Geometry check sheet. Reference: drawing and pictorial views, mm from the part's lowest x, y, z. Give positions to 0.01 mm unless a question says otherwise; leave off trailing zeros. Write each loop counter-clockwise with the first axis right and the second up, starting at its lowest first coordinate (ties: lowest second). Pieces come first, ordered by that corner, then holes. Notation, with made-up numbers: M 68,-13.75 L 80,-13.75 A24 cw 80,21.25 Z; hole C 0.5,-7 d1. An arc over 180 degrees is marked long. Answer as a JSON object with one key per item and string values.
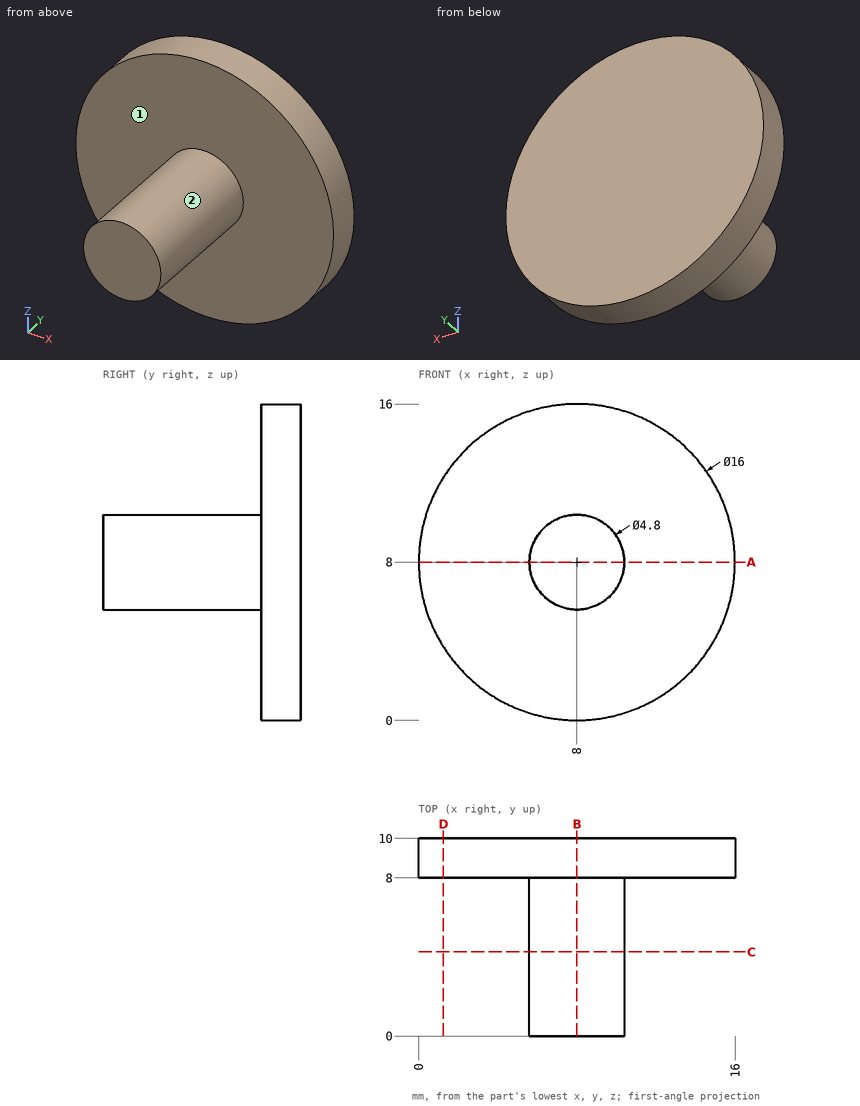
1) Release check for a two-part mould opening along X. For the marked faces 1 and 2 record: pulls with the +X half, pulls with the -X half, needs draft (parallel to the pull), parting line crosses it, or undercut.
Completed:
{"face 1": "needs draft", "face 2": "parting line crosses it"}
2) Section check C-C on y = 4.25. Record the boundary of the cut face in (x, z), and give its area (3 significant figures).
Completed:
{"outline": "C 8,8 d4.8", "area": "18.1 mm2"}
3) Go/stop test with flat-tipped pins: pin 1 (1.5 mm diameter, centred on x = 9, y = 6, fed in from -Z); pin 2 (3 mm diameter, centred on x = 2, z = 8, fed in from -Y); pin 3 (4 mm diameter, centred on x = 10, y = 6.5, fed in from -Z). Record where each tip stops, or that it passes through.
Completed:
{"pin 1": "stops at z = 5.61", "pin 2": "stops at y = 8", "pin 3": "stops at z = 0.03"}
4) Section check B-B on x = 8. Record the boundary of the cut face in (y, z).
Completed:
{"outline": "M 0,5.6 L 8,5.6 L 8,0 L 10,0 L 10,16 L 8,16 L 8,10.4 L 0,10.4 Z"}
5) Thickness scan on L1, parallel to Y at x = 3.5, z = 5.25; L2, parallel to Z at x = 7.75, y = 8.5; L3, parallel to X at y = 9.5, z = 2. Record the ranges inside material, lowest first.
Completed:
{"L1": "y = 8 to 10", "L2": "z = 0 to 16", "L3": "x = 2.71 to 13.29"}
6) Section check D-D on x = 1.25. Record the boundary of the cut face in (y, z), and give its area (3 significant figures).
Completed:
{"outline": "M 8,3.71 L 10,3.71 L 10,12.29 L 8,12.29 Z", "area": "17.2 mm2"}
7) Section check A-A on z = 8. Record the boundary of the cut face in (x, y), and give its area (3 significant figures).
Completed:
{"outline": "M 0,8 L 5.6,8 L 5.6,0 L 10.4,0 L 10.4,8 L 16,8 L 16,10 L 0,10 Z", "area": "70.4 mm2"}
